Check sheet for the modelled part. Datum: model origin and axes. Units: mm. Face numbers are marked on the shaded views. Give positions to 0.01 mm unless a question says otherwise; leave off trailing zeros. Write each loop counter-clockwise with the first axis right and the second up, starting at its lowest first coordinate (ties: lowest second). Pieces come first, ordered by that corner, then holes. Notation, with made-up numbers: (66.25, -3) -> (90.25, -3) arc R22 cw to (90.25, 13) -> close; hole circle Ø4 at (81.25, 51). An arc over 180 degrees is marked (long way). Answer as a JSON object with one key per item and string values.
from build123d import *

# Parameters (mm, degrees)
SCHIZZO1_W                   = 140
SCHIZZO1_H                   = 140
ESTRUSIONE_ESTRUSIONE1_DEPTH = 5
TAGLIO_ESTRUSIONE1_DEPTH     = 159.140950013
TAGLIO_ESTRUSIONE2_DEPTH     = 159.140950013
SCHIZZO4_R                   = 5.5
ESTRUSIONE_ESTRUSIONE2_DEPTH = 2
SMUSSO1_SIZE                 = 2
SCHIZZO5_R                   = 1.75
TAGLIO_ESTRUSIONE3_DEPTH     = 159.21681349


with BuildPart() as part:
    # Schizzo1 → Estrusione-Estrusione1 (new body)
    with BuildSketch(Plane(origin=(0, 0, 0), x_dir=(1, 0, 0), z_dir=(0, 1, 0))):
        with Locations((44.091480444, -39.392386211)):
            Rectangle(SCHIZZO1_W, SCHIZZO1_H)
    extrude(amount=ESTRUSIONE_ESTRUSIONE1_DEPTH)

    # Schizzo2 → Taglio-Estrusione1 (cut, through all)
    with BuildSketch(Plane(origin=(0, 5, 0), x_dir=(1, 0, 0), z_dir=(0, 1, 0))):
        Polygon((-1.159782214, 30.607613789), (-25.908519556, 5.858876448), (-25.908519556, 30.607613789), align=None)
        Polygon((114.091480444, 5.858876448), (89.342743103, 30.607613789), (114.091480444, 30.607613789), align=None)
        Polygon((89.342743103, -109.392386211), (114.091480444, -84.643648869), (114.091480444, -109.392386211), align=None)
        Polygon((-25.908519556, -84.643648869), (-1.159782214, -109.392386211), (-25.908519556, -109.392386211), align=None)
    extrude(amount=-TAGLIO_ESTRUSIONE1_DEPTH, mode=Mode.SUBTRACT)

    # Schizzo3 → Taglio-Estrusione2 (cut, through all)
    with BuildSketch(Plane(origin=(0, 5, 0), x_dir=(1, 0, 0), z_dir=(0, 1, 0))):
        with BuildLine():
            Line((64.984963173, -67.392386211), (23.091480444, -67.392386211))
            ThreePointArc((23.091480444, -67.392386211), (21.591480444, -68.892386211), (23.091480444, -70.392386211))
            Line((23.091480444, -70.392386211), (64.984963173, -70.392386211))
            ThreePointArc((64.984963173, -70.392386211), (66.595257665, -68.892386211), (64.984963173, -67.392386211))
        make_face()
        with BuildLine():
            Line((65.091480444, -8.392386211), (23.091480444, -8.392386211))
            ThreePointArc((23.091480444, -8.392386211), (21.591480444, -9.892386211), (23.091480444, -11.392386211))
            Line((23.091480444, -11.392386211), (65.091480444, -11.392386211))
            ThreePointArc((65.091480444, -11.392386211), (66.591480444, -9.892386211), (65.091480444, -8.392386211))
        make_face()
    extrude(amount=-TAGLIO_ESTRUSIONE2_DEPTH, mode=Mode.SUBTRACT)

    # Schizzo4 → Estrusione-Estrusione2 (add)
    with BuildSketch(Plane(origin=(0, 5, 0), x_dir=(1, 0, 0), z_dir=(0, 1, 0))):
        with Locations(Location((-4.617054872, -88.100921527, 0), (0, 0, 270))):
            Circle(SCHIZZO4_R)
        with Locations(Location((8.817973971, -74.665892685, 0), (0, 0, 270))):
            Circle(SCHIZZO4_R)
        with Locations(Location((-4.617054872, 9.316149105, 0), (0, 0, 270))):
            Circle(SCHIZZO4_R)
        with Locations(Location((8.817973971, -4.118879737, 0), (0, 0, 270))):
            Circle(SCHIZZO4_R)
        with Locations(Location((92.80001576, 9.316149105, 0), (0, 0, 270))):
            Circle(SCHIZZO4_R)
        with Locations(Location((79.364986918, -4.118879737, 0), (0, 0, 270))):
            Circle(SCHIZZO4_R)
        with Locations(Location((92.80001576, -88.100921527, 0), (0, 0, 270))):
            Circle(SCHIZZO4_R)
        with Locations(Location((79.364986918, -74.665892685, 0), (0, 0, 270))):
            Circle(SCHIZZO4_R)
    extrude(amount=ESTRUSIONE_ESTRUSIONE2_DEPTH)

    # Smusso1
    smusso1_edges = [part.edges().sort_by_distance(p)[0] for p in [
        (92.80001576, 7, -14.816149105),
        (79.364986918, 7, -1.381120263),
        (92.80001576, 7, 82.600921527),
        (79.364986918, 7, 69.165892685),
        (-4.617054872, 7, 82.600921527),
        (8.817973971, 7, 69.165892685),
        (-4.617054872, 7, -14.816149105),
        (8.817973971, 7, -1.381120263),
    ]]
    chamfer(smusso1_edges, length=SMUSSO1_SIZE - 0.0001)  # a hair under: the kernel refuses the full size

    # Schizzo5 → Taglio-Estrusione3 (cut, through all)
    with BuildSketch(Plane(origin=(0, 7, 0), x_dir=(1, 0, 0), z_dir=(0, 1, 0))):
        with Locations(Location((-4.617054872, -88.100921527, 0), (0, 0, 270))):
            Circle(SCHIZZO5_R)
        with Locations(Location((8.817973971, -74.665892685, 0), (0, 0, 270))):
            Circle(SCHIZZO5_R)
        with Locations(Location((-4.617054872, 9.316149105, 0), (0, 0, 270))):
            Circle(SCHIZZO5_R)
        with Locations(Location((8.817973971, -4.118879737, 0), (0, 0, 270))):
            Circle(SCHIZZO5_R)
        with Locations(Location((92.80001576, 9.316149105, 0), (0, 0, 270))):
            Circle(SCHIZZO5_R)
        with Locations(Location((79.364986918, -4.118879737, 0), (0, 0, 270))):
            Circle(SCHIZZO5_R)
        with Locations(Location((92.80001576, -88.100921527, 0), (0, 0, 270))):
            Circle(SCHIZZO5_R)
        with Locations(Location((79.364986918, -74.665892685, 0), (0, 0, 270))):
            Circle(SCHIZZO5_R)
    extrude(amount=-TAGLIO_ESTRUSIONE3_DEPTH, mode=Mode.SUBTRACT)


solid = part.part
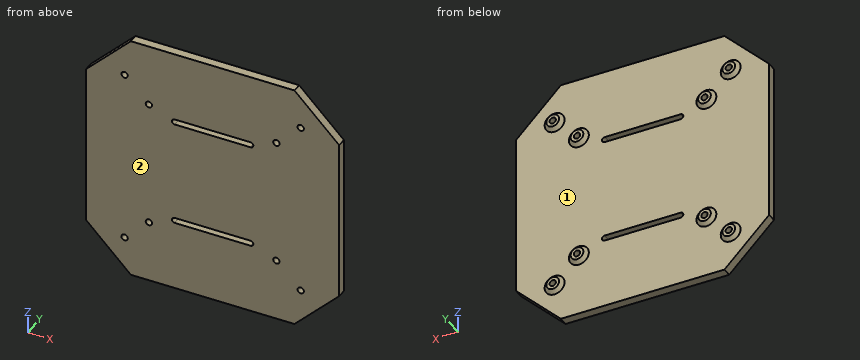
1. Sectioned sample at B-B, the plane z = 23. Enter the section's corners in (x, y).
Determined:
{"outline": "(-25.91, 0) -> (114.09, 0) -> (114.09, 5) -> (-25.91, 5) -> close"}
2. Go/stop test with a flat-tipped pin: P1, Ø10, axis at x = 56.5, z = 72, coming from the +Y side. Record where the tip stops, or that it passes through.
Determined:
{"P1": "y = 5"}
3. Sectioned sample at A-A, the plane y = 2. State how many separate pieces and enclosed holes the cut face has, plus the area to 3 significant figures.
Determined:
{"separate pieces": "1", "enclosed holes": "10", "area": "18,000 mm^2"}
4. Scan lines: L1, parallel to Z at x = 38.5, y = 3.5; L2, parallel to Z at x = 91.5, y = 5.25; L3, parallel to X at y = 5.75, z = 86.5. Record each from-to range of solid material in increasing order. Write a range as [from, to].
Determined:
{"L1": "[-30.61, 8.39], [11.39, 67.39], [70.39, 109.39]", "L2": "[-14.4, -10.49], [-8.14, -4.23], [83.01, 86.93], [89.27, 93.19]", "L3": "[-9.09, -5.32], [-3.91, -0.14], [88.33, 92.09], [93.51, 97.27]"}
5. Mould release check, pull along Z, two halves, no side actions. Record for the marked faces 1 and 2: released by +Z, released by -Z, zero draft, split by the parting line, or undercut.
Determined:
{"face 1": "undercut", "face 2": "zero draft"}
6. Sectioned sample at C-C, the plane x = 69. Enter the section's corners in (y, z).
Determined:
{"outline": "(0, -30.61) -> (5, -30.61) -> (5, 109.39) -> (0, 109.39) -> close"}
